Verification items for the finished model (mm, model axes). Face numbers are marked on the shaded views. A direction names the side the tool comes from. Round coordinates to 2 decimals unless told otherwise and drop trailing zeros. Order: outer loops, then holes, each group sorted by start corner. A loop starts at its lowest first (then second) coordinate and runs counter-clockwise, first axis right, second up. Notation, with made-up numbers: M 69,89.5 L 108,89.5 A23 ccw 108,127.5 Z; hole C 28.25,18.5 d1. An arc over 180 degrees is marked long. Use one line per item in the form item = value. Start each with the question number.
Item 1: Cross-section at B-B on x = 0. Enter the section's corners in (y, z), then the cut area to 3 significant figures.
Item 2: Cross-section at A-A on z = 0. Enter the section's corners in (x, y), then the cut area to 3 significant figures.
Item 3: Go/stop test with flat-tipped pins: pin 1 Ø8 at (y, z) = (-51, -15) entering from +X; pin 2 Ø2 at (y, z) = (-28.5, 1.5) entering from -X (3 decimals); pin 3 Ø8 at (x, z) = (-12.5, -17.5) entering from -Y. Record where each tip stops, or that it passes through.
Item 4: Thickness scan on probe 1 along Y at (x, z) = (8.5, 15); probe 2 along X at (y, z) = (-31, 8.5); probe 3 along X at (y, z) = (-95, -10.5). Record the ranges inside material, lowest first. Write a range as [from, to].
Item 5: Cross-section at C-C on y = -45.5. Enter the section's corners in (x, z).
Item 6: Cross-section at D-D on y = -93.5. Enter the section's corners in (x, z), then the cut area to 3 significant figures.
Item 7: Tool access check on the marked faces 1 and 2. Record the directions out of +Z, -Z, +X, -X, +Y, -Y that give a thin tool (end or side, any length) a straight path to the whole face; none if there is none.
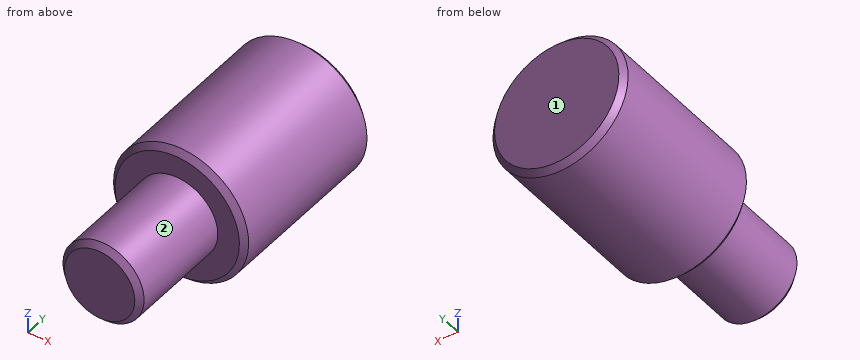
from build123d import *

# Parameters (mm, degrees)
CHAMFER1_SIZE = 2
CHAMFER2_SIZE = 2


with BuildPart() as part:
    # Sketch1 → Revolve1 (revolve)
    with BuildSketch(Plane.XY, mode=Mode.PRIVATE) as revolve1_sk:
        Polygon((0, 0), (25, 0), (25, -65), (15, -65), (15, -105), (0, -105), align=None)
    revolve(revolve1_sk.sketch.rotate(Axis((0, 0, 0), (0, -1, 0)), 90), axis=Axis((0, 0, 0), (0, -1, 0)))

    # Chamfer1
    chamfer1_edges = [part.edges().sort_by_distance(p)[0] for p in [
        (0, -105, -15),
    ]]
    chamfer(chamfer1_edges, length=CHAMFER1_SIZE)

    # Chamfer2
    chamfer2_edges = [part.edges().sort_by_distance(p)[0] for p in [
        (0, -65, -25),
        (0, 0, -25),
    ]]
    chamfer(chamfer2_edges, length=CHAMFER2_SIZE)


solid = part.part
Output values:
q1.outline = M -105,-13 L -103,-15 L -65,-15 L -65,-23 L -63,-25 L -2,-25 L 0,-23 L 0,23 L -2,25 L -63,25 L -65,23 L -65,15 L -103,15 L -105,13 Z
q1.area = 4,440 mm2
q2.outline = M -25,-63 L -23,-65 L -15,-65 L -15,-103 L -13,-105 L 13,-105 L 15,-103 L 15,-65 L 23,-65 L 25,-63 L 25,-2 L 23,0 L -23,0 L -25,-2 Z
q2.area = 4,440 mm2
q3.pin_1 = 22.45
q3.pin_2 = -24.995
q3.pin_3 = -65
q4.probe_1 = [-65, 0]
q4.probe_2 = [-23.51, 23.51]
q4.probe_3 = [-10.71, 10.71]
q5.outline = C 0,0 d50
q6.outline = C 0,0 d30
q6.area = 707 mm2
q7.face_1 = +Z, -Z, +X, -X, +Y
q7.face_2 = -Y
